```python
from build123d import *

# Parameters (mm, degrees)
BOSS_EXTRU_1_DEPTH = 3
CONG_3_R           = 1
CONG_4_R           = 7


with BuildPart() as part:
    # Esquisse1 → Boss.-Extru.1 (new, symmetric)
    with BuildSketch(Plane.XY):
        with BuildLine():
            Line((0, 0), (0, 9))
            Line((0, 9), (1, 9))
            Line((1, 9), (1, 0.09638948))
            Line((1, 0.09638948), (10.121873618, 0.09638948))
            Line((10.121873618, 0.09638948), (70.121873618, 55))
            Line((70.121873618, 55), (70.121873618, 68.436194763))
            Line((70.121873618, 68.436194763), (60.432430442, 68.436194763))
            ThreePointArc((60.432430442, 68.436194763), (52.298183077, 58.663045958), (40.121873618, 55))
            Line((40.121873618, 55), (19.293191489, 55))
            Line((19.293191489, 55), (10.121873618, 55))
            Line((10.121873618, 55), (-4, 55))
            Line((-4, 55), (-4, 40))
            Line((-4, 40), (0, 40))
            Line((0, 40), (0, 49))
            Line((0, 49), (1, 49))
            Line((1, 49), (1, 15))
            Line((1, 15), (-4, 15))
            Line((-4, 15), (-4, 0))
            Line((-4, 0), (0, 0))
        make_face()
    extrude(amount=BOSS_EXTRU_1_DEPTH, both=True)

    # Congé3
    # the kernel refuses this fillet: 1 mm, written as the material it adds along each edge
    with BuildSketch(Plane(origin=(1, 9, -3), x_dir=(0, -1, 0), z_dir=(0, 0, 1)), Plane(origin=(1, 15, -3), x_dir=(-1, 0, 0), z_dir=(0, 0, 1)), Plane(origin=(1, 49, -3), x_dir=(0, -1, 0), z_dir=(0, 0, 1)), Plane(origin=(0, 49, -3), x_dir=(1, 0, 0), z_dir=(0, 0, 1))) as cong_3_piece_1:
        with BuildLine():
            CenterArc((CONG_3_R, -CONG_3_R), CONG_3_R, 90, 90)
            Line((0, -CONG_3_R), (0, 0))
            Line((0, 0), (CONG_3_R, 0))
        make_face()
    extrude(amount=6)
    with BuildSketch(Plane(origin=(0, 9, -3), x_dir=(0, -1, 0), z_dir=(0, 0, 1))) as cong_3_piece_2:
        with BuildLine():
            CenterArc((CONG_3_R, CONG_3_R), CONG_3_R, 180, 90)
            Line((0, CONG_3_R), (0, 0))
            Line((0, 0), (CONG_3_R, 0))
        make_face()
    extrude(amount=6)
    # the kernel refuses this fillet: 1 mm, written as the material it takes off along each edge
    with BuildSketch(Plane(origin=(1, 0.09638948, -5.5), x_dir=(0, 1, 0), z_dir=(0, 0, 1)), Plane(origin=(0, 0, 5.5), x_dir=(0, 1, 0), z_dir=(0, 0, -1)), Plane(origin=(-4, 0, 5.5), x_dir=(1, 0, 0), z_dir=(0, 0, -1)), Plane(origin=(-4, 15, 5.5), x_dir=(0, -1, 0), z_dir=(0, 0, -1)), Plane(origin=(0, 40, -5.5), x_dir=(-1, 0, 0), z_dir=(0, 0, 1)), Plane(origin=(-4, 40, -5.5), x_dir=(0, 1, 0), z_dir=(0, 0, 1)), Plane(origin=(-4, 55, -5.5), x_dir=(1, 0, 0), z_dir=(0, 0, 1))) as cong_3_2_piece_1:
        with BuildLine():
            CenterArc((CONG_3_R, -CONG_3_R), CONG_3_R, 90, 90)
            Line((0, -CONG_3_R), (0, 0))
            Line((0, 0), (CONG_3_R, 0))
        make_face()
    extrude(amount=11, mode=Mode.SUBTRACT)

    # Congé4
    # the kernel refuses this fillet: 7 mm, written as the material it takes off along each edge
    with BuildSketch(Plane(origin=(10.121873618, 0.09638948, -9.798414872), x_dir=(-1, 0, 0), z_dir=(0, 0, 1))) as cong_4_piece_1:
        with BuildLine():
            CenterArc((CONG_4_R * 0.388480849828, -CONG_4_R), CONG_4_R, 90, 42.460390035)
            Line((-CONG_4_R * 0.286599498638, -CONG_4_R * 0.262255787474), (0, 0))
            Line((0, 0), (CONG_4_R * 0.388480849828, 0))
        make_face()
    extrude(amount=19.596829744, mode=Mode.SUBTRACT)
    with BuildSketch(Plane(origin=(70.121873618, 55, -10.707405636), x_dir=(-0.7377442125256176, -0.6750803484659854, 0), z_dir=(0, 0, 1))) as cong_4_piece_2:
        with BuildLine():
            CenterArc((CONG_4_R * 0.440423179223, -CONG_4_R), CONG_4_R, 90, 47.539609965)
            Line((-CONG_4_R * 0.297321033302, -CONG_4_R * 0.324919651534), (0, 0))
            Line((0, 0), (CONG_4_R * 0.440423179223, 0))
        make_face()
    extrude(amount=21.414811273, mode=Mode.SUBTRACT)
    with BuildSketch(Plane(origin=(70.121873618, 68.436194763, -20.5), x_dir=(0, -1, 0), z_dir=(0, 0, 1))) as cong_4_piece_3:
        with BuildLine():
            CenterArc((CONG_4_R, -CONG_4_R), CONG_4_R, 90, 90)
            Line((0, -CONG_4_R), (0, 0))
            Line((0, 0), (CONG_4_R, 0))
        make_face()
    extrude(amount=41, mode=Mode.SUBTRACT)
    with BuildSketch(Plane(origin=(60.432430442, 68.436194763, -13.492760312), x_dir=(1, 0, 0), z_dir=(0, 0, 1))) as cong_4_piece_4:
        with BuildLine():
            CenterArc((4.197104125, -7), CONG_4_R, 90, 57.467043301)
            ThreePointArc((-1.704471625, -3.235507515), (-0.785102058, -1.653119949), (0, 0))
            Line((0, 0), (4.197104125, 0))
        make_face()
    extrude(amount=26.985520624, mode=Mode.SUBTRACT)


solid = part.part
```
The listing builds one solid part. Answer for the finished solid, in the listing's coordinates (mm). A direction names the side the tool comes from. Give positions to 0.01 mm unless a question says otherwise; leave off trailing zeros. Loops run counter-clockwise (first coordinate to the right, second up) from the corner with the lowest first, then second, coordinate; pieces in that order, holes last. Notation, with made-up numbers: M 42.25,15 L 83.25,15 A19 ccw 83.25,43 Z; hole C 12.25,65.25 d6. An arc over 180 degrees is marked long. One line per item, written item: value.
Q1. A cutting plane is placed at A-A on y = 6.5. Determine the outline of the cut face in (x, z).
Working result:
outline: M -4,-3 L 0,-3 L 0,3 L -4,3 Z; M 1,-3 L 17.12,-3 L 17.12,3 L 1,3 Z
Q2. Find the intervals of material crossed by line 1 (X direction, y = 48, z = -0.75); line 2 (X direction, y = 40.5, z = -2.5); line 3 (Y direction, x = 5, z = -1.5), in increasing order. Write a range as from..to.
Working result:
line 1: x = -4..0, 1..62.47
line 2: x = -3.87..-0.13, 1..54.28
line 3: y = 0.1..55
Q3. Flat-ended cylindrical pins translate along their axes: P1, Ø3, axis at y = 37.5, z = 0.5, coming from the -X side; P2, Ø1.8, axis at y = 4.5, z = -1, coming from the +X side; P3, Ø1.5, axis at y = 56, z = 1.5, coming from the +X side; P4, Ø0.6, axis at x = -2, z = -1, coming from the -Y side. Find the tip coordinate at first contact, or state that the pin passes through.
Working result:
P1: stops at x = 1
P2: stops at x = 15.92
P3: stops at x = 69.99
P4: stops at y = 0
Q4. Determine the mould class of faces 1 (the face through (1, 5, 0)), 2 (the face through (-2, 0, 0)), 3 (the face through (69.5, 55.2, 0)), 4 (the face through (1, 32, 0)) for opening direction X: +X half, -X half, draft (parallel to the pull), parting line (faces both ways), or undercut.
Working result:
face 1: undercut
face 2: draft
face 3: +X half
face 4: undercut
Q5. A cutting plane is placed at C-C on y = 57. Determine the outline of the cut face in (x, z), then the cut area to 3 significant figures.
Working result:
outline: M 49.3,-3 L 70.04,-3 L 70.04,3 L 49.3,3 Z
area: 124 mm^2
Q6. For faces 5 (the face through (-1, 15, 0)), 6 (the face through (5, 0.096, 0)), 7 (the face through (0, 44, 0)), determine the directions among +Z, -Z, +X, -X, +Y, -Y from which every point of the face is accessible in a straight line to the end or side of a thin tool.
Working result:
face 5: +Z, -Z, -X
face 6: +Z, -Z, +X, -Y
face 7: +Z, -Z
Q7. A cutting plane is placed at D-D on x = 56.5. Determine the outline of the cut face in (y, z).
Working result:
outline: M 42.54,-3 L 62.28,-3 L 62.28,3 L 42.54,3 Z
